Check sheet for the modelled part. Datum: model origin and axes. Units: mm. A direction names the side the tool comes from. Coordinates: 2 decimals unless noted, no trailing zeros.
from build123d import *

# Parameters (mm, degrees)
SKETCH1_R           = 6.14
BOSS_EXTRUDE1_DEPTH = 1
BOSS_EXTRUDE2_START = -18
SKETCH1_7_R         = 6.14
SKETCH1_7_W         = 59
SKETCH1_7_H         = 32
SKETCH1_7_W_2       = 56
SKETCH1_7_H_2       = 29
BOSS_EXTRUDE2_DEPTH = 18
BOSS_EXTRUDE4_DEPTH = 14
FILLET1_R           = 1
CUT_EXTRUDE2_DEPTH  = 14
CUT_EXTRUDE3_DEPTH  = 14
FILLET2_R           = 1
SKETCH24_W          = 56
SKETCH24_H          = 1.5
CUT_EXTRUDE5_DEPTH  = 4
BOSS_EXTRUDE5_REACH = 54.785
SKETCH26_W          = 2
SKETCH26_H          = 1.85
BOSS_EXTRUDE6_REACH = 72.258
SKETCH27_W          = 2
SKETCH27_H          = 1.85
SKETCH29_W          = 8
SKETCH29_H          = 5
CUT_EXTRUDE7_DEPTH  = 10
CHAMFER1_SIZE       = 0.5
CHAMFER2_SIZE       = 0.25


# Some blends are built 0.0001 mm under size
with BuildPart() as part:
    # Sketch1 → Boss-Extrude1 (new body)
    with BuildSketch(Plane(origin=(0, 0, 0), x_dir=(1, 0, 0), z_dir=(0, 1, 0))):
        with BuildLine():
            Line((26.916456077, -7.14), (8.050130866, 27.948393818))
            ThreePointArc((8.050130866, 27.948393818), (0, 32.76), (-8.050130866, 27.948393818))
            Line((-8.050130866, 27.948393818), (-26.916456077, -7.14))
            Line((-26.916456077, -7.14), (-29.5, -7.14))
            Line((-29.5, -7.14), (-29.5, -39.14))
            Line((-29.5, -39.14), (29.5, -39.14))
            Line((29.5, -39.14), (29.5, -7.14))
            Line((29.5, -7.14), (26.916456077, -7.14))
        make_face()
        with Locations(Location((-12.7, 0, 0), (0, 0, 270))):
            Circle(SKETCH1_R, mode=Mode.SUBTRACT)
        with Locations(Location((0, 23.62, 0), (0, 0, 270))):
            Circle(SKETCH1_R, mode=Mode.SUBTRACT)
        with Locations(Location((12.7, 0, 0), (0, 0, 270))):
            Circle(SKETCH1_R, mode=Mode.SUBTRACT)
    extrude(amount=BOSS_EXTRUDE1_DEPTH)

    # Sketch1<7> → Boss-Extrude2 (add)
    # profile 1 of 4: a face of its own
    with BuildSketch(Plane(origin=(0, 0, 0), x_dir=(1, 0, 0), z_dir=(0, 1, 0)).offset(BOSS_EXTRUDE2_START)):
        with Locations(Location((-12.7, 0, 0), (0, 0, 270))):
            Circle(SKETCH1_7_R)
    # profile 2 of 4: a face of its own
    with BuildSketch(Plane(origin=(0, 0, 0), x_dir=(1, 0, 0), z_dir=(0, 1, 0)).offset(BOSS_EXTRUDE2_START)):
        with Locations(Location((0, 23.62, 0), (0, 0, 270))):
            Circle(SKETCH1_7_R)
    # profile 3 of 4: a face of its own
    with BuildSketch(Plane(origin=(0, 0, 0), x_dir=(1, 0, 0), z_dir=(0, 1, 0)).offset(BOSS_EXTRUDE2_START)):
        with Locations(Location((12.7, 0, 0), (0, 0, 270))):
            Circle(SKETCH1_7_R)
    # profile 4 of 4: a face of its own
    with BuildSketch(Plane(origin=(0, 0, 0), x_dir=(1, 0, 0), z_dir=(0, 1, 0)).offset(BOSS_EXTRUDE2_START)):
        with Locations((0, -23.14)):
            Rectangle(SKETCH1_7_W, SKETCH1_7_H)
        with Locations((0, -23.14)):
            Rectangle(SKETCH1_7_W_2, SKETCH1_7_H_2, mode=Mode.SUBTRACT)
    extrude(amount=BOSS_EXTRUDE2_DEPTH)


with BuildPart() as boss_extrude2_kept_piece:
    # of the separate pieces the step leaves, the one the design keeps (boss_extrude2_pieces_kept)
    add(part.part.solids().sort_by_distance((26.916456077, 0, 7.14))[0])

    # Sketch16 → Boss-Extrude4 (add)
    with BuildSketch(Plane.XZ):
        with BuildLine():
            Line((-24.645685539, 7.14), (-6.288614265, -27.001261692))
            ThreePointArc((-6.288614265, -27.001261692), (0, -30.76), (6.288614265, -27.001261692))
            Line((6.288614265, -27.001261692), (24.645685539, 7.14))
            Line((24.645685539, 7.14), (26.916456077, 7.14))
            Line((26.916456077, 7.14), (8.050130866, -27.948393818))
            ThreePointArc((8.050130866, -27.948393818), (0, -32.76), (-8.050130866, -27.948393818))
            Line((-8.050130866, -27.948393818), (-26.916456077, 7.14))
            Line((-26.916456077, 7.14), (-24.645685539, 7.14))
        make_face()
    extrude(amount=BOSS_EXTRUDE4_DEPTH)

    # Fillet1
    fillet1_edges = [boss_extrude2_kept_piece.edges().sort_by_distance(p)[0] for p in [
        (-29.5, -8.5, 7.14),
        (29.5, -8.5, 7.14),
        (29.5, -8.5, 39.14),
        (-29.5, -8.5, 39.14),
    ]]
    fillet(fillet1_edges, radius=FILLET1_R)

    # Sketch19 → Cut-Extrude2 (cut)
    with BuildSketch(Plane(origin=(29.5, 0, 0), x_dir=(0, 0, -1), z_dir=(1, 0, 0))):
        with BuildLine():
            Line((-27.24, -1), (-19.04, -1))
            ThreePointArc((-19.04, -1), (-18.757157288, -1.117157288), (-18.64, -1.4))
            Line((-18.64, -1.4), (-18.64, -4.6))
            ThreePointArc((-18.64, -4.6), (-18.757157288, -4.882842712), (-19.04, -5))
            Line((-19.04, -5), (-27.24, -5))
            ThreePointArc((-27.24, -5), (-27.522842712, -4.882842712), (-27.64, -4.6))
            Line((-27.64, -4.6), (-27.64, -1.4))
            ThreePointArc((-27.64, -1.4), (-27.522842712, -1.117157288), (-27.24, -1))
        make_face()
    extrude(amount=-CUT_EXTRUDE2_DEPTH, mode=Mode.SUBTRACT)

    # Sketch21 → Cut-Extrude3 (cut)
    with BuildSketch(Plane.XY.offset(8.64)):
        Polygon((8, 0), (-8, 0), (-8, -5.911265283), (-8, -14), (8, -14), (8, -5.911265283), align=None)
    extrude(amount=-CUT_EXTRUDE3_DEPTH, mode=Mode.SUBTRACT)

    # Fillet2
    fillet2_edges = [boss_extrude2_kept_piece.edges().sort_by_distance(p)[0] for p in [
        (0, 1, 39.14),
        (-29.5, 1, 23.14),
        (29.5, 1, 23.14),
        (-27.708228038, 1, 7.14),
        (29.207106781, 1, 7.432893219),
        (29.207106781, 1, 38.847106781),
        (-29.207106781, 1, 7.432893219),
        (-29.207106781, 1, 38.847106781),
        (27.708228038, 1, 7.14),
        (17.483293471, 1, -10.404196909),
        (0, 1, -32.76),
        (-17.483293471, 1, -10.404196909),
        (-12.7, 1, -6.14),
        (0, 1, -29.76),
        (12.7, 1, -6.14),
    ]]
    fillet(fillet2_edges, radius=FILLET2_R - 0.0001)  # a hair under: the kernel refuses the full size

    # Sketch24 → Cut-Extrude5 (cut)
    with BuildSketch(Plane(origin=(0, -18, 0), x_dir=(-1, 0, 0), z_dir=(0, -1, 0))):
        with Locations((0, -7.89)):
            Rectangle(SKETCH24_W, SKETCH24_H)
    extrude(amount=-CUT_EXTRUDE5_DEPTH, mode=Mode.SUBTRACT)

    # Sketch26 → Boss-Extrude5 (add, up to next)
    with BuildSketch(Plane(origin=(0, 0, 7.14), x_dir=(-1, 0, 0), z_dir=(0, 0, -1)), mode=Mode.PRIVATE) as boss_extrude5_sk1:
        with Locations((27, -17.075)):
            Rectangle(SKETCH26_W, SKETCH26_H)
    boss_extrude5_tool1 = extrude(boss_extrude5_sk1.sketch, amount=-BOSS_EXTRUDE5_REACH, mode=Mode.PRIVATE) - boss_extrude2_kept_piece.part
    # Sketch26 → Boss-Extrude5 (add, up to next)
    with BuildSketch(Plane(origin=(0, 0, 7.14), x_dir=(-1, 0, 0), z_dir=(0, 0, -1)), mode=Mode.PRIVATE) as boss_extrude5_sk2:
        with Locations((-27, -17.075)):
            Rectangle(SKETCH26_W, SKETCH26_H)
    boss_extrude5_tool2 = extrude(boss_extrude5_sk2.sketch, amount=-BOSS_EXTRUDE5_REACH, mode=Mode.PRIVATE) - boss_extrude2_kept_piece.part
    add(boss_extrude5_tool1.solids().sort_by_distance((-27, -17.075, 7.14))[0])
    add(boss_extrude5_tool2.solids().sort_by_distance((27, -17.075, 7.14))[0])

    # Sketch27 → Boss-Extrude6 (add, up to next)
    with BuildSketch(Plane.ZY.offset(-26), mode=Mode.PRIVATE) as boss_extrude6_sk1:
        with Locations((36.64, -17.075)):
            Rectangle(SKETCH27_W, SKETCH27_H)
    boss_extrude6_tool1 = extrude(boss_extrude6_sk1.sketch, amount=BOSS_EXTRUDE6_REACH, mode=Mode.PRIVATE) - boss_extrude2_kept_piece.part
    add(boss_extrude6_tool1.solids().sort_by_distance((26, -17.075, 36.64))[0])

    # Sketch29 → Cut-Extrude7 (cut)
    with BuildSketch(Plane.XZ.offset(14)):
        with Locations((0, -32.034355417)):
            Rectangle(SKETCH29_W, SKETCH29_H)
    extrude(amount=-CUT_EXTRUDE7_DEPTH, mode=Mode.SUBTRACT)

    # Chamfer1
    # the kernel refuses this chamfer: 0.5, 0.374030712 mm, written as the material it takes off along each edge
    with BuildSketch(Plane(origin=(-4, -4, -31.838247988), x_dir=(-0.89007215049111, 0, 0.4558196649116082), z_dir=(0, -1, 0))) as chamfer1_piece_1:
        with BuildLine():
            Line((0.371500885, 0), (CHAMFER1_SIZE * 0.455819664912, -CHAMFER1_SIZE * 0.890072150491))
            Line((CHAMFER1_SIZE * 0.455819664912, -CHAMFER1_SIZE * 0.890072150491), (0, 0))
            ThreePointArc((0, 0), (0.18881851, 0.001887165), (0.371500885, 0))
        make_face()
    extrude(amount=11.285841494, mode=Mode.SUBTRACT)
    with BuildSketch(Plane(origin=(4, -4, -31.838247988), x_dir=(0.8900721504911105, 0, 0.4558196649116072), z_dir=(0, -1, 0))) as chamfer1_piece_2:
        with BuildLine():
            Line((0.371500885, 0), (CHAMFER1_SIZE * 0.455819664912, CHAMFER1_SIZE * 0.890072150491))
            Line((CHAMFER1_SIZE * 0.455819664912, CHAMFER1_SIZE * 0.890072150491), (0, 0))
            ThreePointArc((0, 0), (0.18881851, -0.001887165), (0.371500885, 0))
        make_face()
    extrude(amount=11.285841494, mode=Mode.SUBTRACT)

    # Chamfer2
    chamfer2_edges = [boss_extrude2_kept_piece.edges().sort_by_distance(p)[0] for p in [
        (28, -15.075, 7.14),
        (-28, -15.075, 7.14),
        (-27, -16.15, 7.14),
        (27, -16.15, 7.14),
    ]]
    chamfer(chamfer2_edges, length=CHAMFER2_SIZE)


solid = boss_extrude2_kept_piece.part
(1) Scan lines: line 1 along X through (y, z) = (-4.5, 8); line 2 along X through (y, z) = (0.05, 0); line 3 along X through (y, z) = (-10.25, 35.5). Record each from-to range of solid material in increasing order.
(2) Gauge pin test, flat ends, axial feed: P1, Ø3, axis at x = -18.5, z = 11, coming from the -Y side; P2, Ø0.8, axis at x = 28.5, y = -4, coming from the -Z side; P3, Ø10, axis at y = -7, z = 3.5, coming from the -X side; P4, Ø1, axis at y = -8, z = 1.5, coming from the -X side. Record the tip position at first contact, or that the pin passes through.
(3) Section check C-C, the plane z = 0. Count the separate pieces of the cut face and the enclosed holes in it, plus the area to 3 significant figures.
(4) Set-up check for faces 5 (the face through (0, -9, 39.14)), 6 (the face through (-8, -7, 8)), 7 (the face through (29, -1, 23)), 8 (the face through (0, -8, 37.64)), 9 (the face through (0, -4, -31)): record each of +Z, -Z, +X, -X, +Y, -Y from which the full face is reachable in a straight line by a thin tool's end or side.
(5) Draft check along Y on faces 1 (the face through (-17.35, -6.9, -10.65)), 2 (the face through (29, -5, 23)), 3 (the face through (-28, -8, 23)), 4 (the face through (2, -18, 36)). Enter one of: pulls with the +Y half, pulls with the -Y half, needs draft (parallel to the pull), parting line crosses it, or undercut.
Determined:
1. line 1: x = -29.49 to -8, 8 to 29.49
1. line 2: x = -23.08 to -18.84, -6.56 to 6.56, 18.84 to 23.08
1. line 3: x = -29.5 to -28, 28 to 29.5
2. P1: stops at y = 0
2. P2: stops at z = 7.14
2. P3: stops at x = -29.5
2. P4: stops at x = -24.15
3. separate pieces: 3
3. enclosed holes: 0
3. area: 83.8 mm2
4. face 5: +Z, +X, -X, +Y, -Y
4. face 6: -Y
4. face 7: +X
4. face 8: none
4. face 9: -Z, -Y
5. face 1: needs draft
5. face 2: undercut
5. face 3: undercut
5. face 4: pulls with the -Y half
